Part model, mm, in its own coordinate system. Face numbers are marked on the shaded views. A direction names the side the tool comes from. Round coordinates to 2 decimals unless told otherwise and drop trailing zeros. Loops run counter-clockwise (first coordinate to the right, second up) from the corner with the lowest first, then second, coordinate; pieces in that order, holes last. Notation, with made-up numbers: M 85,43 L 113,43 A28 cw 113,70 Z; hole C -21,-21.5 d9. An arc over 180 degrees is marked long. Put each result on its own line as item: value. Start each with the question number.
1) Which spindle directions (+Z, -Z, +X, -X, +Y, -Y) get a long thin tool onto all of the face, cutting with end or side? Do the marked faces 4 and 5. Say none if no direction does.
2) Slice it at B-B on y = 181. Give the cut face in (x, z), then the cut area to 3 significant figures.
3) Pull direction Z, two halves, no side cores. Call the marked faces 1, 2 and 3: +Z half, -Z half, draft (parallel to the pull), parting line (faces both ways), or undercut.
4) Drop a flat-ended pin along its axis: pin 1 Ø2 at (y, z) = (149.5, 11) entering from +X. Give the stop position or say it passes through.
5) Slice it at A-A on x = 7.5. Give the cut face in (y, z), then the cut area to 3 significant figures.
6) Probe line 1 along Z through (x, y) = (-11, 112); line 2 along Z through (x, y) = (-17, 245); line 3 along X through (y, z) = (74.5, 31.5). List the from-to ranges inside material, lowest first.
7) Slice it at C-C on z = 24.5. Give the cut face in (x, y).
Solid Edge part; units mm, degrees
sketch "Sketch1" plane through (0, 0, 0) normal (0, -1, 0) x (1, 0, 0)
  line L0 (20, 36) -> (-16, 36)
  line L1 (-16, 36) -> (-16, -36)
  line L2 (-16, -36) -> (20, -36)
  line L3 (20, -36) -> (20, -40)
  line L4 (20, -40) -> (-20, -40)
  line L5 (-20, -40) -> (-20, 40)
  line L6 (-20, 40) -> (20, 40)
  line L7 (20, 40) -> (20, 36)
  dimension "D1" = 20
  dimension "D2" = 20
  dimension "D3" = 20
extrude "Protrusion1" add sketch "Sketch1" against normal blind 350
sketch "Sketch2" plane through (0, 175, 40) normal (0, 0, 1) x (0, 1, 0)
  line L0 (-175, 20) -> (-135, -20)
extrude "Cutout1" cut sketch "Sketch2" against normal through all material side at (0.0354, 19.9646, 40)
sketch "Sketch3" plane through (0, 175, 40) normal (0, 0, 1) x (0, 1, 0)
  line L0 (175, 20) -> (135, -20)
extrude "Cutout2" cut sketch "Sketch3" against normal through all material side at (0.0354, 330.0354, 40)
hole "Bohrung_1" at (-16, 142.5, 17) direction (-1, 0, 0) diameter 5.5 end up to next
hole "Hole1" at (-16, 207.5, 17) direction (-1, 0, 0) diameter 5.5 end up to next
hole "Bohrung_3" at (-16, 50, 15.6) direction (-1, 0, 0) diameter 4.5 end up to next
hole "Hole2" at (-16, 105, 15.6) direction (-1, 0, 0) diameter 4.5 end up to next
hole "Hole3" at (-16, 245, 15.6) direction (-1, 0, 0) diameter 4.5 end up to next
hole "Hole4" at (-16, 300, 15.6) direction (-1, 0, 0) diameter 4.5 end up to next
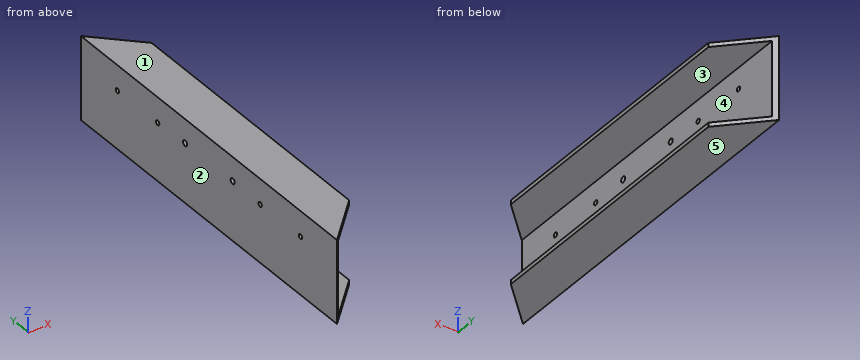
Recorded:
1. face 4: +X, +Y, -Y
1. face 5: -Z, +X, -X, +Y, -Y
2. outline: M -20,-40 L 20,-40 L 20,-36 L -16,-36 L -16,36 L 20,36 L 20,40 L -20,40 Z
2. area: 608 mm2
3. face 1: +Z half
3. face 2: draft
3. face 3: undercut
4. pin 1: stops at x = -16
5. outline: M 27.5,-40 L 322.5,-40 L 322.5,-36 L 27.5,-36 Z; M 27.5,36 L 322.5,36 L 322.5,40 L 27.5,40 Z
5. area: 2,360 mm2
6. line 1: z = -40 to -36, 36 to 40
6. line 2: z = -40 to 13.35, 17.85 to 40
6. line 3: x = -20 to -16
7. outline: M -20,0 L -16,4 L -16,346 L -20,350 Z
